The model under review builds one solid part; all positions refer to its coordinate system, in mm. Face numbers are marked on the shaded views. A direction names the side the tool comes from. Round coordinates to 2 decimals unless told otherwise and drop trailing zeros. Loops run counter-clockwise (first coordinate to the right, second up) from the corner with the lowest first, then second, coordinate; pieces in that order, holes last. Notation, with made-up numbers: M 6,88.25 L 11,88.25 A21 ccw 11,113.25 Z; hole C 74.5,-15.75 d7. An arc over 180 degrees is marked long. Return JSON: item names as keys, results as strings. Group by question number.
Q1. Consider section A-A (z = 0). State the section outline as (x, y) points.
Q2. Consider section D-D (y = 3). Count the separate pieces of the cut face and the enclosed holes in it, and give its area (3 significant figures).
Q3. Consider section B-B (x = 7). State the section outline as (y, z) points (3 decimals), and give its area (3 significant figures).
Q4. To check wall thickness, follow line 1 along X through (y, z) = (5, 0); line 2 along Z through (x, y) = (-11, 2) (3 decimals); line 3 along Z through (x, y) = (-5.5, 4) (3 decimals). State the ranges of each line that lie inside material, in increasing order.
Q5. Draft analysis for pull direction X (two halves, no side actions). For the marked faces 1, 2 and 3, state which applies: pulls with the +X half, pulls with the -X half, needs draft (parallel to the pull), parting line crosses it, or undercut.
Q6. Clearance check with flat-ended pins moving along their axes: pin 1 Ø1 at (y, z) = (1, 6) entering from -X; pin 2 Ø3 at (x, y) = (-2, 2) entering from -Z; pin 3 Ø1 at (x, y) = (-3.5, 1.5) entering from +Z. State where each tip first meets the part, or that it passes through.
Q7. For the marked faces 4, 5, 6 and 7, list the 3-axis set-ups (+Z, -Z, +X, -X, +Y, -Y) from which the entire face can be reached by the end or side of a thin tool; tool diameter is ignored.
Q8. Consider section C-C (x = 1.5). State the section outline as (y, z) points (3 decimals).
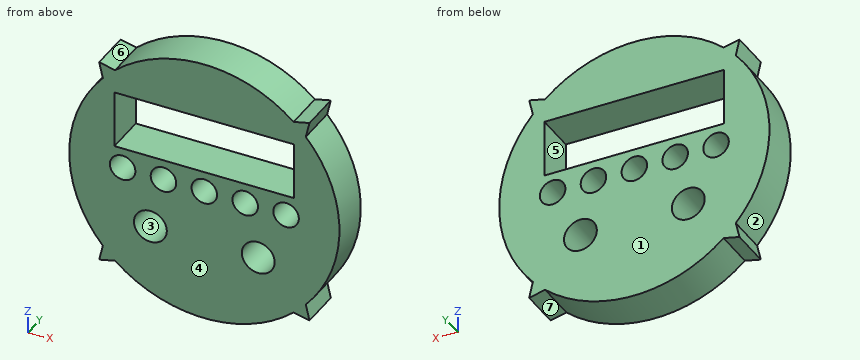
from build123d import *

# Parameters (mm, degrees)
SKETCH1_R           = 1.984375
SKETCH1_R_2         = 2.5527
SKETCH1_W           = 27.94
SKETCH1_H           = 8.89
BOSS_EXTRUDE1_DEPTH = 6.35


with BuildPart() as part:
    # Sketch1 → Boss-Extrude1 (new body)
    with BuildSketch(Plane(origin=(0, 0, 0), x_dir=(1, 0, 0), z_dir=(0, 1, 0))):
        with BuildLine():
            Line((13.870085237, 15.767711804), (16.343875029, 16.343875029))
            Line((16.343875029, 16.343875029), (15.767711804, 13.870085237))
            ThreePointArc((15.767711804, 13.870085237), (21, 0), (15.767711804, -13.870085237))
            Line((15.767711804, -13.870085237), (16.343875029, -16.343875029))
            Line((16.343875029, -16.343875029), (13.870085237, -15.767711804))
            ThreePointArc((13.870085237, -15.767711804), (0, -21), (-13.870085237, -15.767711804))
            Line((-13.870085237, -15.767711804), (-16.343875029, -16.343875029))
            Line((-16.343875029, -16.343875029), (-15.767711804, -13.870085237))
            ThreePointArc((-15.767711804, -13.870085237), (-21, 0), (-15.767711804, 13.870085237))
            Line((-15.767711804, 13.870085237), (-16.343875029, 16.343875029))
            Line((-16.343875029, 16.343875029), (-13.870085237, 15.767711804))
            ThreePointArc((-13.870085237, 15.767711804), (0, 21), (13.870085237, 15.767711804))
        make_face()
        with Locations(Location((-12.7, 0, 0), (0, 0, 270))):
            Circle(SKETCH1_R, mode=Mode.SUBTRACT)
        with Locations(Location((-6.35, 0, 0), (0, 0, 270))):
            Circle(SKETCH1_R, mode=Mode.SUBTRACT)
        with Locations(Location((0, 0, 0), (0, 0, 270))):
            Circle(SKETCH1_R, mode=Mode.SUBTRACT)
        with Locations(Location((-8.382, 8.382, 0), (0, 0, 270))):
            Circle(SKETCH1_R_2, mode=Mode.SUBTRACT)
        with Locations(Location((8.382, 8.382, 0), (0, 0, 270))):
            Circle(SKETCH1_R_2, mode=Mode.SUBTRACT)
        with Locations(Location((6.35, 0, 0), (0, 0, 270))):
            Circle(SKETCH1_R, mode=Mode.SUBTRACT)
        with Locations(Location((12.7, 0, 0), (0, 0, 270))):
            Circle(SKETCH1_R, mode=Mode.SUBTRACT)
        with Locations((0, -7.62)):
            Rectangle(SKETCH1_W, SKETCH1_H, mode=Mode.SUBTRACT)
    extrude(amount=BOSS_EXTRUDE1_DEPTH)


solid = part.part
Values:
{
 "1": {"outline": "M -21,0 L -14.68,0 L -14.68,6.35 L -21,6.35 Z; M -10.72,0 L -8.33,0 L -8.33,6.35 L -10.72,6.35 Z; M -4.37,0 L -1.98,0 L -1.98,6.35 L -4.37,6.35 Z; M 1.98,0 L 4.37,0 L 4.37,6.35 L 1.98,6.35 Z; M 8.33,0 L 10.72,0 L 10.72,6.35 L 8.33,6.35 Z; M 14.68,0 L 21,0 L 21,6.35 L 14.68,6.35 Z"},
 "2": {"separate pieces": "1", "enclosed holes": "8", "area": "1,050 mm2"},
 "3": {"outline": "M 0,-19.799 L 6.35,-19.799 L 6.35,-10.528 L 0,-10.528 Z; M 0,-6.236 L 6.35,-6.236 L 6.35,-1.875 L 0,-1.875 Z; M 0,1.875 L 6.35,1.875 L 6.35,3.175 L 0,3.175 Z; M 0,12.065 L 6.35,12.065 L 6.35,19.799 L 0,19.799 Z", "area": "144 mm2"},
 "4": {"line 1": "x = -21 to -14.68, -10.72 to -8.33, -4.37 to -1.98, 1.98 to 4.37, 8.33 to 10.72, 14.68 to 21", "line 2": "z = -17.889 to -1.024, 1.024 to 3.175, 12.065 to 17.889", "line 3": "z = -20.267 to -1.793, 1.793 to 3.175, 12.065 to 20.267"},
 "5": {"face 1": "needs draft", "face 2": "pulls with the -X half", "face 3": "undercut"},
 "6": {"pin 1": "stops at x = -20.27", "pin 2": "stops at z = -20.99", "pin 3": "stops at z = 20.78"},
 "7": {"face 4": "+Z, -Z, +X, -X, -Y", "face 5": "+Y, -Y", "face 6": "+Z, +Y, -Y", "face 7": "-Z, +Y, -Y"},
 "8": {"outline": "M 0,-20.946 L 6.35,-20.946 L 6.35,-1.299 L 0,-1.299 Z; M 0,1.299 L 6.35,1.299 L 6.35,3.175 L 0,3.175 Z; M 0,12.065 L 6.35,12.065 L 6.35,20.946 L 0,20.946 Z"}
}
